Geometry check sheet. Reference: the model listing, model coordinates, mm. A direction names the side the tool comes from. Round coordinates to 2 decimals unless told otherwise and drop trailing zeros. Write each loop counter-clockwise with the first axis right and the second up, starting at its lowest first coordinate (ties: lowest second). Pieces come first, ordered by that corner, then holes.
Item 1: Cross-section at A-A (z = 1.8). Enter the section's corners in (x, y).
Item 2: Access from +Z, -Z, +X, -X, +Y, -Y to the whole of each face (thin tool, end or side, straight path). Record for faces 1 (the face through (-30, -7.5, 1)), 2 (the face through (-40, 5, 1)), 3 (the face through (-1, 7.5, 1)), 4 (the face through (39, 5, 1)), 5 (the face through (23, -7.5, 1)).
Item 3: Cross-section at C-C (x = 1). Enter the section's corners in (y, z), then the cut area to 3 significant figures.
Item 4: Scan lines: probe 1 along Y at (x, z) = (12, 1.7); probe 2 along X at (y, z) = (-5.5, 1.25); probe 3 along X at (y, z) = (-31.5, 1.3). Record each from-to range of solid material in increasing order.
Item 5: Depth check by flat-ended pin: P1, Ø1.5, axis at x = -40, z = 2, coming from the +Y side; P2, Ø0.8, axis at y = -5.5, z = 1, coming from the -X side; P3, Ø0.9, axis at x = 40, z = 1, coming from the -Y side. Enter the tip coordinate at first touch or a pass-through.
Item 6: Cross-section at B-B (y = -21). Enter the section's corners in (x, z), then the cut area to 3 significant figures.
from build123d import *

# Parameters (mm, degrees)
ESBO_O1_W                = 76
ESBO_O1_H                = 15
ESBO_O1_W_2              = 20
ESBO_O1_H_2              = 30
ESBO_O1_W_3              = 3
ESBO_O1_H_3              = 10
RESSALTO_EXTRUS_O1_DEPTH = 3
FILETE1_R                = 5


with BuildPart() as part:
    # Esboço1 → Ressalto-extrusão1 (new body)
    with BuildSketch(Plane.XY):
        Rectangle(ESBO_O1_W, ESBO_O1_H)
        with Locations((-7, -22.5)):
            Rectangle(ESBO_O1_W_2, ESBO_O1_H_2)
        with Locations((39.5, 0)):
            Rectangle(ESBO_O1_W_3, ESBO_O1_H_3)
        with Locations((-39.5, 0)):
            Rectangle(ESBO_O1_W_3, ESBO_O1_H_3)
    extrude(amount=RESSALTO_EXTRUS_O1_DEPTH)

    # Filete1
    filete1_edges = [part.edges().sort_by_distance(p)[0] for p in [
        (3, -7.5, 1.5),
        (3, -37.5, 1.5),
        (-17, -37.5, 1.5),
        (-17, -7.5, 1.5),
    ]]
    fillet(filete1_edges, radius=FILETE1_R)


solid = part.part
Resolved:
1. outline: (-41, -5) - (-38, -5) - (-38, -7.5) - (-22, -7.5) arc R5 cw to (-17, -12.5) - (-17, -32.5) arc R5 ccw to (-12, -37.5) - (-2, -37.5) arc R5 ccw to (3, -32.5) - (3, -12.5) arc R5 cw to (8, -7.5) - (38, -7.5) - (38, -5) - (41, -5) - (41, 5) - (38, 5) - (38, 7.5) - (-38, 7.5) - (-38, 5) - (-41, 5) - close
2. face 1: +Z, -Z, -X, -Y
2. face 2: +Z, -Z, -X, +Y
2. face 3: +Z, -Z, +X, -X, +Y
2. face 4: +Z, -Z, +X, +Y
2. face 5: +Z, -Z, +X, -Y
3. outline: (-36.5, 0) - (7.5, 0) - (7.5, 3) - (-36.5, 3) - close
3. area: 132 mm2
4. probe 1: y = -7.5 to 7.5
4. probe 2: x = -38 to 38
4. probe 3: x = -17 to 3
5. P1: stops at y = 5
5. P2: stops at x = -38
5. P3: stops at y = -5
6. outline: (-17, 0) - (3, 0) - (3, 3) - (-17, 3) - close
6. area: 60.0 mm2
